from build123d import *

# Parameters (mm, degrees)
F0_W     = 128
F0_H     = 340
F1_DEPTH = 245
F2_SIZE2 = 20
F2_SIZE  = 5
F3_W     = 18
F3_H     = 40
F4_DEPTH = 50
F7_R     = 5


with BuildPart() as f1:
    # F0 (on Top) → F1 (new body)
    with BuildSketch(Plane.XY):
        with Locations((64, 170)):
            Rectangle(F0_W, F0_H)
    extrude(amount=F1_DEPTH)

    # F2
    f2_edges = [f1.edges().sort_by_distance(p)[0] for p in [
        (128, 0, 122.5),
        (0, 0, 122.5),
        (64, 0, 245),
    ]]
    f2_side = f1.faces().sort_by_distance((64, 0, 122.5))[0]
    chamfer(f2_edges, length=F2_SIZE, length2=F2_SIZE2, reference=f2_side)

    # F3 (on face) → F4 (join)
    with BuildSketch(Plane(origin=(0, 340, 0), x_dir=(-1, 0, 0), z_dir=(0, 1, 0))):
        with Locations((-94, 195)):
            Rectangle(F3_W, F3_H)
    extrude(amount=F4_DEPTH)

    # F8: sweep along a path in F6
    with BuildLine(Plane.XY.offset(195)) as f8_path:
        Line((94, 390), (94, 395))
        ThreePointArc((94, 395), (88.1421356237, 409.1421356237), (74, 415))
        Line((74, 415), (34, 415))
    # F7 (on face) → F8 (sweep)
    with BuildSketch(Plane(origin=(0, 390, 0), x_dir=(-1, 0, 0), z_dir=(0, 1, 0))):
        with Locations((-94, 195)):
            Circle(F7_R)
    sweep(path=f8_path.line)


solid = f1.part
Here's how the part is built. I have some questions about the finished solid (model axes, mm). A direction names the side the tool comes from. Give positions to 0.01 mm unless a question says otherwise; leave off trailing zeros. Order: outer loops, then holes, each group sorted by start corner. A loop starts at its lowest first (then second) coordinate and runs counter-clockwise, first axis right, second up. Notation, with made-up numbers: M 56,-13.75 L 69,-13.75 A10 cw 69,-1.75 Z; hole C 6,-20.75 d7. An arc over 180 degrees is marked long. Answer as a JSON object with one key per item and string values. Group by question number.
1) I'm going to push flat-ended pins straight in: pin 1 Ø14.5 at (x, y) = (90.5, 367) entering from -Z; pin 2 Ø1.5 at (x, z) = (94.5, 92) entering from +Y; pin 3 Ø12 at (y, z) = (370.5, 188) entering from +X. Where does each tip first touch, or does it pass through?
2) We'd pull the mould along Y, two halves only. Please class faces 4 (the flat face through (128, 178, 121)), 5 (the cylindrical face through (53.72, 410.23, 196.5)), 6 (the flat face through (63.104, 10.14, 242.535)): pulls with the +Y half, pulls with the -Y half, needs draft (parallel to the pull), parting line crosses it, or undercut.
3) Suppose I cut it at A-A, the plane z = 195. Write out the boundary of the cut face in (x, y).
4) Suppose I cut it at B-B, the plane x = 43. Write out the boundary of the cut face in (y, z), plus the area to 3 significant figures.
5) Please list where these lines run through material, in increasing order: L1, parallel to Y at x = 78, z = 162; L2, parallel to Z at x = 86, y = 360.5. Write a range as [from, to].
6) Suppose I cut it at C-C, the plane x = 10. Write out the boundary of the cut face in (y, z), plus the area to 4 significant figures.
7) On a 3-axis mill with a long thin cutter (end or side, diameter ignored), from which of +Z, -Z, +X, -X, +Y, -Y can I reach the whole of each face in a straight line? I mean faces 1 (the flat face through (96, 390, 200)), 2 (the flat face through (103, 365, 195)), 3 (the flat face through (94, 365, 175)). Say none if no direction works.
8) Suppose I cut it at D-D, the plane y = 381.5. Write out the boundary of the cut face in (x, z), plus the area to 3 significant figures.
Results found:
{
 "1": {"pin 1": "z = 175", "pin 2": "y = 340", "pin 3": "x = 103"},
 "2": {"face 4": "needs draft", "face 5": "undercut", "face 6": "pulls with the -Y half"},
 "3": {"outline": "M 0,20 L 5,0 L 123,0 L 128,20 L 128,340 L 103,340 L 103,390 L 99,390 L 99,395 A25 ccw 74,420 L 34,420 L 34,410 L 74,410 A15 cw 89,395 L 89,390 L 85,390 L 85,340 L 0,340 Z"},
 "4": {"outline": "M 0,0 L 340,0 L 340,245 L 20,245 L 0,240 Z; C 415,195 d10", "area": "83,300 mm²"},
 "5": {"L1": "[0, 340]", "L2": "[175, 215]"},
 "6": {"outline": "M 0,0 L 340,0 L 340,245 L 20,245 L 0,240 Z", "area": "83,250 mm²"},
 "7": {"face 1": "none", "face 2": "+Z, -Z, +X, +Y", "face 3": "-Z, +X, -X, +Y"},
 "8": {"outline": "M 85,175 L 103,175 L 103,215 L 85,215 Z", "area": "720 mm²"}
}
